Read the model definition and answer for the solid it produces. Units are mm, in the model's axes. A direction names the side the tool comes from. Give positions to 0.01 mm unless a question says otherwise; leave off trailing zeros. Order: outer loops, then holes, each group sorted by start corner. A loop starts at its lowest first (then second) coordinate and runs counter-clockwise, first axis right, second up. Notation, with made-up numbers: (40, 41.25) - (89, 41.25) arc R22 cw to (89, 73.25) - close; hole circle Ø6 at (-16, 3.5). An arc over 180 degrees is marked (long way). Return JSON: item names as keys, results as strings.
```python
from build123d import *

# Parameters (mm, degrees)
F0_W     = 50.8
F0_H     = 38.1
F1_DEPTH = 88.9
F2_R     = 3.048
F3_T     = -2.54


with BuildPart() as f1:
    # F0 (on Top) → F1 (new body)
    with BuildSketch(Plane.XY):
        with Locations((25.4, 19.05)):
            Rectangle(F0_W, F0_H)
    extrude(amount=F1_DEPTH)

    # F2
    f2_edges = [f1.edges().sort_by_distance(p)[0] for p in [
        (0, 0, 44.45),
        (0, 38.1, 44.45),
    ]]
    fillet(f2_edges, radius=F2_R)

    # F3
    f3_openings = [f1.faces().sort_by_distance(p)[0] for p in [
        (25.451031, 19.05, 0),
    ]]
    offset(amount=F3_T, openings=f3_openings)


solid = f1.part
```
Q1. Consider L1, parallel to Y at x = 14, z = 47; L2, parallel to X at y = 33, z = 42; L3, parallel to Z at x = 37, y = 21.5. Determine where each line is inside the solid, lowest interval first.
Values:
{"L1": "y = 0 to 2.54, 35.56 to 38.1", "L2": "x = 0 to 2.54, 48.26 to 50.8", "L3": "z = 86.36 to 88.9"}
Q2. Given pin 1 (3 mm diameter, centred on x = 41, y = 12, fed in from -Z), flat-ended and moving along its own axis, determine where the tip first touches the part or whether it passes through.
Values:
{"pin 1": "stops at z = 86.36"}
Q3. For faces 4 (the flat face through (27, 38.1, 44)), 5 (the flat face through (48.26, 19, 43)), determine the directions among +Z, -Z, +X, -X, +Y, -Y from which every point of the face is accessible in a straight line to the end or side of a thin tool.
Values:
{"face 4": "+Z, -Z, +X, -X, +Y", "face 5": "-Z"}
Q4. Determine the mould class of faces 1 (the flat face through (0, 19, 44)), 2 (the cylindrical face through (0.869, 0.917, 45.072)), 3 (the flat face through (25, 35.56, 43)) for opening direction Y: released by +Y, released by -Y, zero draft, split by the parting line, or undercut.
Values:
{"face 1": "zero draft", "face 2": "released by -Y", "face 3": "undercut"}
Q5. A cutting plane is placed at B-B (y = 6.5). Write down the section's boundary in (x, z), and give its area (3 significant figures).
Values:
{"outline": "(0, 0) - (2.54, 0) - (2.54, 86.36) - (48.26, 86.36) - (48.26, 0) - (50.8, 0) - (50.8, 88.9) - (0, 88.9) - close", "area": "568 mm²"}
Q6. A cutting plane is placed at A-A (z = 48.5). Write down the section's boundary in (x, y).
Values:
{"outline": "(0, 3.05) arc R3.05 ccw to (3.05, 0) - (50.8, 0) - (50.8, 38.1) - (3.05, 38.1) arc R3.05 ccw to (0, 35.05) - close; hole (2.54, 3.05) arc R0.51 ccw to (3.05, 2.54) - (48.26, 2.54) - (48.26, 35.56) - (3.05, 35.56) arc R0.51 ccw to (2.54, 35.05) - close"}
Q7. A cutting plane is placed at C-C (x = 9.5). Write down the section's boundary in (y, z).
Values:
{"outline": "(0, 0) - (2.54, 0) - (2.54, 86.36) - (35.56, 86.36) - (35.56, 0) - (38.1, 0) - (38.1, 88.9) - (0, 88.9) - close"}
